```python
from build123d import *

# Parameters (mm, degrees)
BOSS_EXTRUDE1_DEPTH = 6.35
FILLET1_R           = 6.35
SKETCH2_W           = 50.8
SKETCH2_H           = 6.35
BOSS_EXTRUDE2_DEPTH = 19.05
SKETCH3_W           = 50.8
SKETCH3_H           = 6.35
BOSS_EXTRUDE3_DEPTH = 38.1
SKETCH4_W           = 50.8
SKETCH4_H           = 6.35
BOSS_EXTRUDE4_DEPTH = 63.5
FILLET2_R           = 2.54
SKETCH5_R           = 5
SKETCH5_W           = 73.66
SKETCH5_H           = 11.43
CUT_EXTRUDE3_DEPTH  = 284.408566149
SKETCH6_R           = 3.175
CUT_EXTRUDE4_DEPTH  = 284.408566149
SKETCH8_R           = 3.175
CUT_EXTRUDE5_DEPTH  = 284.408566149
CUT_EXTRUDE6_DEPTH  = 180.280400037


with BuildPart() as part:
    # Sketch1 → Boss-Extrude1 (new body)
    with BuildSketch(Plane.XY):
        with BuildLine():
            add(Edge.make_bspline(
                [(-276.130119323, 8.693130358), (-231.459725957, 13.892182525), (-160.606907467, 22.045765928), (-55.21857633, 32.848239562), (-5.484684229, 39.5878223), (20.294760191, 40.734135472), (52.215253795, 43.311195196), (77.433370096, 43.854837121), (107.657853328, 39.590984865), (131.131357877, 34.766526999), (149.499224412, 30.294140301), (163.418705178, 23.059137739), (171.530279946, 16.921852673), (175.269753602, 13.29140622)],
                knots=[0, 0, 0, 0, 0.247403676, 0.462108507, 0.504395118, 0.627983171, 0.653401948, 0.743134379, 0.818760812, 0.882434425, 0.924179622, 0.96050512, 1, 1, 1, 1], degree=3))
            add(Edge.make_bspline(
                [(-276.130119323, 8.693130358), (-174.260953063, 0.911239157), (-23.669401798, 0.683864032), (127.515095646, 0.681371654), (175.269753602, 13.29140622)],
                knots=[0, 0, 0, 0, 0.67646369, 1, 1, 1, 1], degree=3))
        make_face()
    extrude(amount=BOSS_EXTRUDE1_DEPTH)

    # Fillet1
    fillet1_edges = [part.edges().sort_by_distance(p)[0] for p in [
        (175.269753602, 13.29140622, 3.175),
    ]]
    fillet(fillet1_edges, radius=FILLET1_R)

    # Sketch2 → Boss-Extrude2 (add, symmetric)
    with BuildSketch(Plane(origin=(0, 0, 0), x_dir=(1, 0, 0), z_dir=(0, 1, 0))):
        with Locations((-149.130119323, -3.175)):
            Rectangle(SKETCH2_W, SKETCH2_H)
        with Locations((40.537724966, -3.175)):
            Rectangle(SKETCH2_W, SKETCH2_H)
    extrude(amount=BOSS_EXTRUDE2_DEPTH, both=True)

    # Sketch3 → Boss-Extrude3 (add)
    with BuildSketch(Plane(origin=(0, 0, 0), x_dir=(1, 0, 0), z_dir=(0, 1, 0))):
        with Locations((-149.130119323, -3.175)):
            Rectangle(SKETCH3_W, SKETCH3_H)
    extrude(amount=BOSS_EXTRUDE3_DEPTH)

    # Sketch4 → Boss-Extrude4 (add)
    with BuildSketch(Plane(origin=(0, 0, 0), x_dir=(1, 0, 0), z_dir=(0, 1, 0))):
        with Locations((40.537724966, -3.175)):
            Rectangle(SKETCH4_W, SKETCH4_H)
    extrude(amount=BOSS_EXTRUDE4_DEPTH)

    # Fillet2
    fillet2_edges = [part.edges().sort_by_distance(p)[0] for p in [
        (65.937724966, 0.882409675, 3.175),
        (15.137724966, 0.715325792, 3.175),
        (-123.730119323, 1.809475424, 3.175),
        (-174.530119323, 3.18492072, 3.175),
        (-174.530119323, 20.264304266, 3.175),
        (-123.730119323, 25.734914395, 3.175),
        (15.137724966, 40.575893827, 3.175),
        (65.937724966, 43.322928246, 3.175),
        (65.937724966, -19.05, 3.175),
        (15.137724966, -19.05, 3.175),
        (-174.530119323, -19.05, 3.175),
        (-123.730119323, -19.05, 3.175),
        (-174.530119323, 38.1, 3.175),
        (-123.730119323, 38.1, 3.175),
        (65.937724966, 63.5, 3.175),
        (15.137724966, 63.5, 3.175),
    ]]
    fillet(fillet2_edges, radius=FILLET2_R)

    # Sketch5 → Cut-Extrude3 (cut, through all)
    with BuildSketch(Plane.XY):
        with Locations(Location((140.241842338, 17.410004614, 0), (0, 0, 180))):
            Circle(SKETCH5_R)
        with Locations(Location((-23.613557662, 17.410004614, 0), (0, 0, 180))):
            Circle(SKETCH5_R)
        with Locations((27.973842338, 19.812)):
            Rectangle(SKETCH5_W, SKETCH5_H)
    extrude(amount=CUT_EXTRUDE3_DEPTH, mode=Mode.SUBTRACT)

    # Sketch6 → Cut-Extrude4 (cut, through all)
    with BuildSketch(Plane.XY):
        with Locations(Location((55.777724966, 53.34, 0), (0, 0, 180))):
            Circle(SKETCH6_R)
        with Locations(Location((25.297724966, 53.34, 0), (0, 0, 180))):
            Circle(SKETCH6_R)
        with Locations(Location((55.777724966, -8.89, 0), (0, 0, 180))):
            Circle(SKETCH6_R)
        with Locations(Location((25.297724966, -8.89, 0), (0, 0, 180))):
            Circle(SKETCH6_R)
        with Locations(Location((-133.890119323, 30.48, 0), (0, 0, 180))):
            Circle(SKETCH6_R)
        with Locations(Location((-164.370119323, 30.48, 0), (0, 0, 180))):
            Circle(SKETCH6_R)
        with Locations(Location((-133.890119323, -8.89, 0), (0, 0, 180))):
            Circle(SKETCH6_R)
        with Locations(Location((-164.370119323, -8.89, 0), (0, 0, 180))):
            Circle(SKETCH6_R)
    extrude(amount=CUT_EXTRUDE4_DEPTH, mode=Mode.SUBTRACT)

    # Sketch8 → Cut-Extrude5 (cut, through all)
    with BuildSketch(Plane(origin=(0, 0, 0), x_dir=(-1, 0, 0), z_dir=(0, 0, -1))):
        with BuildLine():
            Line((152.305119323, 35.56), (152.305119323, 22.652979968))
            Line((152.305119323, 22.652979968), (145.955119323, 2.430574079))
            Line((145.955119323, 2.430574079), (145.955119323, -16.51))
            ThreePointArc((145.955119323, -16.51), (145.211170547, -18.306051224), (143.415119323, -19.05))
            Line((143.415119323, -19.05), (171.990119323, -19.05))
            ThreePointArc((171.990119323, -19.05), (173.786170547, -18.306051224), (174.530119323, -16.51))
            Line((174.530119323, -16.51), (174.530119323, 0.732669408))
            add(Edge.make_bspline(
                [(174.530119323, 0.732669408), (174.530119323, 0.827098892), (174.534332017, 0.922829058), (174.542975148, 1.019550557), (174.556231365, 1.116913443), (174.574237139, 1.214535389), (174.647171539, 1.525872583), (174.720530405, 1.739086636), (174.817987929, 1.947258959), (174.939041393, 2.145669731), (175.081636695, 2.329900504), (175.40320955, 2.663115508), (175.582254784, 2.812169869), (175.77623684, 2.94020009), (175.980813085, 3.044996297), (176.191284552, 3.125888304), (176.499832231, 3.209844277), (176.59675239, 3.231309016), (176.693582493, 3.24801799), (176.789935606, 3.260093994), (176.885455508, 3.26770712), (176.979825307, 3.271063977)],
                knots=[0, 0, 0, 0, 0, 0, 0, 0.156541714, 0.156541714, 0.156541714, 0.156541714, 0.156541714, 0.5, 0.5, 0.5, 0.5, 0.5, 0.843458286, 0.843458286, 0.843458286, 0.843458286, 0.843458286, 1, 1, 1, 1, 1, 1, 1], degree=6))
            add(Edge.make_bspline(
                [(276.130119323, 8.693130358), (243.083160763, 6.168638939), (210.036144296, 4.446920485), (176.979825307, 3.271063977)],
                knots=[0, 0, 0, 0, 0.219448812, 0.219448812, 0.219448812, 0.219448812], degree=3))
            add(Edge.make_bspline(
                [(276.130119323, 8.693130358), (241.143309206, 12.765139518), (210.289343773, 16.325674302), (176.792020475, 20.015402476)],
                knots=[0, 0, 0, 0, 0.193771865, 0.193771865, 0.193771865, 0.193771865], degree=3))
            add(Edge.make_bspline(
                [(176.792020475, 20.015402476), (176.702534659, 20.025259334), (176.612334841, 20.039047045), (176.521708613, 20.056916996), (176.430972739, 20.078987549), (176.340465644, 20.105336292), (176.052123832, 20.203632982), (175.856494206, 20.292258021), (175.667511078, 20.402173666), (175.489198081, 20.532546831), (175.325208173, 20.681273314), (175.070618463, 20.965445878), (174.972096017, 21.093854031), (174.883813086, 21.22927413), (174.806550855, 21.370274525), (174.740735934, 21.515302785), (174.633101241, 21.807741296), (174.590880763, 21.955079167), (174.559863739, 22.103342362), (174.539790441, 22.251097449), (174.530119323, 22.397057265), (174.530119323, 22.540132369)],
                knots=[0, 0, 0, 0, 0, 0, 0, 0.155935083, 0.155935083, 0.155935083, 0.155935083, 0.155935083, 0.499997058, 0.499997058, 0.499997058, 0.499997058, 0.499997058, 0.752183878, 0.752183878, 0.752183878, 0.752183878, 0.752183878, 1, 1, 1, 1, 1, 1, 1], degree=6))
            Line((174.530119323, 22.540132369), (174.530119323, 35.56))
            ThreePointArc((174.530119323, 35.56), (173.786170547, 37.356051224), (171.990119323, 38.1))
            Line((171.990119323, 38.1), (149.765119323, 38.1))
            ThreePointArc((149.765119323, 38.1), (151.561170547, 37.356051224), (152.305119323, 35.56))
        make_face()
        with Locations((164.370119323, -8.89)):
            Circle(SKETCH8_R, mode=Mode.SUBTRACT)
        with Locations((164.370119323, 30.48)):
            Circle(SKETCH8_R, mode=Mode.SUBTRACT)
    extrude(amount=-CUT_EXTRUDE5_DEPTH, mode=Mode.SUBTRACT)

    # Sketch10 → Cut-Extrude6 (cut, through all)
    with BuildSketch(Plane(origin=(0, 0, 0), x_dir=(-1, 0, 0), z_dir=(0, 0, -1))):
        with BuildLine():
            Line((-95.157002323, 17.295971295), (-95.157002323, 1.810619129))
            add(Edge.make_bspline(
                [(-95.157002323, 1.810619129), (-98.122222912, 1.963522837), (-101.08564833, 2.137394625), (-104.047002323, 2.335082223)],
                knots=[0.821015806, 0.821015806, 0.821015806, 0.821015806, 0.840729968, 0.840729968, 0.840729968, 0.840729968], degree=3))
            Line((-104.047002323, 2.335082223), (-104.047002323, 17.295971295))
            ThreePointArc((-104.047002323, 17.295971295), (-99.602002323, 21.740971295), (-95.157002323, 17.295971295))
        make_face()
    extrude(amount=-CUT_EXTRUDE6_DEPTH, mode=Mode.SUBTRACT)


solid = part.part
```
Here's how the part is built. I have some questions about the finished solid (model axes, mm). A direction names the side the tool comes from. Give positions to 0.01 mm unless a question says otherwise; leave off trailing zeros. Order: outer loops, then holes, each group sorted by start corner. A loop starts at its lowest first (then second) coordinate and runs counter-clockwise, first axis right, second up. Notation, with made-up numbers: M 67.5,-26 L 112.5,-26 A22 cw 112.5,11 Z; hole C -6,26 d5. An arc over 180 degrees is marked long. Use a Markdown table: item, result. Add a question column.
1. For pin 1 Ø1 at (y, z) = (47.5, 4) entering from -X; pin 2 Ø5 at (x, y) = (25.3, 53.34) entering from -Z; pin 3 Ø1.9 at (y, z) = (-7.5, 2) entering from +X; pin 4 Ø3 at (y, z) = (-7.5, 5) entering from -X, each with a flat end and sliding along its axis, tell me the tip position at first contact or that it passes through.
2. Suppose I cut it at C-C (z = 4.25). Give the number of separate pieces and of enclosed holes in the cut face, and give its area (3 significant figures).
3. If we mould it in two halves opening along X, with no side actions, what happens to faces 4 (the flat face through (40, 63.5, 3)), 5 (the flat face through (-149.175, 12.683, 3.131)), 6 (the flat face through (104.047, 10, 3))? For each: +X half, -X half, draft (parallel to the pull), parting line (faces both ways), or undercut.
4. On a 3-axis mill with a long thin cutter (end or side, diameter ignored), from which of +Z, -Z, +X, -X, +Y, -Y can I reach the whole of each face in a straight line? I mean faces 1 (the flat face through (5.4, 13.6, 0)), 2 (the flat face through (27, 14.097, 3)), 3 (the flat face through (95.157, 10, 3)). Say none if no direction works.
5. Suppose I cut it at A-A (y = -8.89). List the corners of the cut face in (x, z) for me.
6. Suppose I cut it at B-B (y = 53.34). List the corners of the cut face in (x, z) for me.
7. I need wall thicknesses on probe 1 along X at (y, z) = (53.34, 1.5); probe 2 along X at (y, z) = (-8.89, 3); probe 3 along Y at (x, z) = (12, 3.75). Which ranges of each line are inside material? Lowest first, please. Write a range as from..to.
Results list:
| question | item | result |
|---|---|---|
| 1 | pin 1 | stops at x = 15.14 |
| 1 | pin 2 | passes through |
| 1 | pin 3 | stops at x = 65.94 |
| 1 | pin 4 | stops at x = -145.96 |
| 2 | separate pieces | 1 |
| 2 | enclosed holes | 9 |
| 2 | area | 12,000 mm² |
| 3 | face 4 | draft |
| 3 | face 5 | -X half |
| 3 | face 6 | undercut |
| 4 | face 1 | -Z, +X, -X, +Y, -Y |
| 4 | face 2 | +Z, -Z |
| 4 | face 3 | +Z, -Z, -Y |
| 5 | outline | M -145.96,0 L -137.07,0 L -137.07,6.35 L -145.96,6.35 Z; M -130.72,0 L -123.73,0 L -123.73,6.35 L -130.72,6.35 Z; M 15.14,0 L 22.12,0 L 22.12,6.35 L 15.14,6.35 Z; M 28.47,0 L 52.6,0 L 52.6,6.35 L 28.47,6.35 Z; M 58.95,0 L 65.94,0 L 65.94,6.35 L 58.95,6.35 Z |
| 6 | outline | M 15.14,0 L 22.12,0 L 22.12,6.35 L 15.14,6.35 Z; M 28.47,0 L 52.6,0 L 52.6,6.35 L 28.47,6.35 Z; M 58.95,0 L 65.94,0 L 65.94,6.35 L 58.95,6.35 Z |
| 7 | probe 1 | x = 15.14..22.12, 28.47..52.6, 58.95..65.94 |
| 7 | probe 2 | x = -145.96..-137.07, -130.72..-123.73, 15.14..22.12, 28.47..52.6, 58.95..65.94 |
| 7 | probe 3 | y = 0.72..14.1, 25.53..40.37 |
